Source: CAD feature listing. Evaluate the final solid. Frame: model axes, mm. A direction names the side the tool comes from. Give positions to 0.01 mm unless a question says otherwise; leave off trailing zeros. Loops run counter-clockwise (first coordinate to the right, second up) from the corner with the lowest first, then second, coordinate; pieces in that order, holes last.
```python
from build123d import *

# Parameters (mm, degrees)
SKETCH_1_W          = 40
SKETCH_1_H          = 39
EXTRUDE_1_DEPTH     = 20
SKETCH_2_W          = 20
SKETCH_2_H          = 2
EXTRUDE_2_DEPTH     = 8
SKETCH_3_W          = 20
SKETCH_3_H          = 2
EXTRUDE_3_DEPTH     = 8
CUT_EXTRUDE_3_REACH = 62.539
SKETCH_4_R          = 2
CUT_EXTRUDE_5_REACH = 62.539
SKETCH_5_R          = 2
SKETCH_7_R          = 3
EXTRUDE_5_DEPTH     = 0.5
SKETCH_9_R          = 1.5
EXTRUDE_6_DEPTH     = 5
FILLET_7_R          = 1
FILLET_8_R          = 1
FILLET_9_R          = 1
FILLET_10_R         = 1


# Read off the part's stored shape, not the designer's step: #4-40 机械螺纹 螺柱3
with BuildPart() as part:
    # 草图1 → 凸台-拉伸1 (new body)
    with BuildSketch(Plane(origin=(0, 0, 0), x_dir=(0, 0, -1), z_dir=(1, 0, 0))):
        with Locations((20, 19.5)):
            Rectangle(SKETCH_1_W, SKETCH_1_H)
    extrude(amount=EXTRUDE_1_DEPTH)

    # 草图2 → 凸台-拉伸2 (add)
    with BuildSketch(Plane.XY):
        with Locations((10, 30)):
            Rectangle(SKETCH_2_W, SKETCH_2_H)
    extrude(amount=EXTRUDE_2_DEPTH)

    # 草图3 → 凸台-拉伸3 (add)
    with BuildSketch(Plane(origin=(0, 0, -40), x_dir=(-1, 0, 0), z_dir=(0, 0, -1))):
        with Locations((-10, 30)):
            Rectangle(SKETCH_3_W, SKETCH_3_H)
    extrude(amount=EXTRUDE_3_DEPTH)

    # 草图4 → 切除-拉伸3 (cut, up to next)
    with BuildSketch(Plane(origin=(0, 31, 0), x_dir=(1, 0, 0), z_dir=(0, 1, 0)), mode=Mode.PRIVATE) as cut_extrude_3_sk1:
        with Locations(Location((5, -4, 0), (0, 0, 180))):
            Circle(SKETCH_4_R)
    cut_extrude_3_tool1 = extrude(cut_extrude_3_sk1.sketch, amount=-CUT_EXTRUDE_3_REACH, mode=Mode.PRIVATE) & part.part
    # 草图4 → 切除-拉伸3 (cut, up to next)
    with BuildSketch(Plane(origin=(0, 31, 0), x_dir=(1, 0, 0), z_dir=(0, 1, 0)), mode=Mode.PRIVATE) as cut_extrude_3_sk2:
        with Locations(Location((15, -4, 0), (0, 0, 180))):
            Circle(SKETCH_4_R)
    cut_extrude_3_tool2 = extrude(cut_extrude_3_sk2.sketch, amount=-CUT_EXTRUDE_3_REACH, mode=Mode.PRIVATE) & part.part
    add(cut_extrude_3_tool1.solids().sort_by_distance((5, 31, 4))[0], mode=Mode.SUBTRACT)
    add(cut_extrude_3_tool2.solids().sort_by_distance((15, 31, 4))[0], mode=Mode.SUBTRACT)

    # 草图5 → 切除-拉伸5 (cut, up to next)
    with BuildSketch(Plane(origin=(0, 31, 0), x_dir=(1, 0, 0), z_dir=(0, 1, 0)), mode=Mode.PRIVATE) as cut_extrude_5_sk1:
        with Locations(Location((5, 44, 0), (0, 0, 270))):
            Circle(SKETCH_5_R)
    cut_extrude_5_tool1 = extrude(cut_extrude_5_sk1.sketch, amount=-CUT_EXTRUDE_5_REACH, mode=Mode.PRIVATE) & part.part
    # 草图5 → 切除-拉伸5 (cut, up to next)
    with BuildSketch(Plane(origin=(0, 31, 0), x_dir=(1, 0, 0), z_dir=(0, 1, 0)), mode=Mode.PRIVATE) as cut_extrude_5_sk2:
        with Locations(Location((15, 44, 0), (0, 0, 270))):
            Circle(SKETCH_5_R)
    cut_extrude_5_tool2 = extrude(cut_extrude_5_sk2.sketch, amount=-CUT_EXTRUDE_5_REACH, mode=Mode.PRIVATE) & part.part
    add(cut_extrude_5_tool1.solids().sort_by_distance((5, 31, -44))[0], mode=Mode.SUBTRACT)
    add(cut_extrude_5_tool2.solids().sort_by_distance((15, 31, -44))[0], mode=Mode.SUBTRACT)

    # 草图7 → 凸台-拉伸5 (add)
    with BuildSketch(Plane(origin=(0, 39, 0), x_dir=(1, 0, 0), z_dir=(0, 1, 0))):
        with Locations(Location((10, 10, 0), (0, 0, 90))):
            Circle(SKETCH_7_R)
    extrude(amount=EXTRUDE_5_DEPTH)

    # 草图9 → 凸台-拉伸6 (add)
    with BuildSketch(Plane(origin=(0, 39, 0), x_dir=(1, 0, 0), z_dir=(0, 1, 0))):
        with Locations(Location((10, 10, 0), (0, 0, 270))):
            Circle(SKETCH_9_R)
    extrude(amount=EXTRUDE_6_DEPTH)

    # 圆角7
    fillet_7_edges = [part.edges().sort_by_distance(p)[0] for p in [
        (20, 39, -20),
        (0, 35, -40),
        (20, 35, -40),
        (20, 35, 0),
        (0, 39, -20),
        (0, 35, 0),
        (10, 39, 0),
        (10, 39, -40),
    ]]
    fillet(fillet_7_edges, radius=FILLET_7_R)

    # 圆角8
    fillet_8_edges = [part.edges().sort_by_distance(p)[0] for p in [
        (20, 30, 8),
        (0, 30, 8),
    ]]
    fillet(fillet_8_edges, radius=FILLET_8_R)

    # 圆角9
    fillet_9_edges = [part.edges().sort_by_distance(p)[0] for p in [
        (0, 30, -48),
        (20, 30, -48),
    ]]
    fillet(fillet_9_edges, radius=FILLET_9_R)

    # #4-40 机械螺纹 螺柱3 outline → #4-40 机械螺纹 螺柱3 (revolve, cut)
    with BuildSketch(Plane(origin=(10, 0, -10), x_dir=(1, 0, 0), z_dir=(0, 0, 1))):
        Polygon((1.5, 44), (1.04394, 44), (1.4224, 43.62154), (1.4224, 39.5), (1.5, 39.5), align=None)
    revolve(axis=Axis((10, 0, -10), (0, 1, 0)), mode=Mode.SUBTRACT)

    # 圆角10
    fillet_10_edges = [part.edges().sort_by_distance(p)[0] for p in [
        (20, 14.5, -40),
        (0, 14.5, 0),
        (20, 14.5, 0),
        (0, 14.5, -40),
    ]]
    fillet(fillet_10_edges, radius=FILLET_10_R)


solid = part.part
```
(1) Section A-A, the plane x = 5. Return the cut outline in (y, z), then the cut area to 3 significant figures.
A:
outline: (0, -40) - (29, -40) - (29, -42) - (31, -42) - (31, -40) - (38, -40) arc R1 ccw to (39, -39) - (39, -1) arc R1 ccw to (38, 0) - (31, 0) - (31, 2) - (29, 2) - (29, 0) - (0, 0) - close; (29, -48) - (31, -48) - (31, -46) - (29, -46) - close; (29, 6) - (31, 6) - (31, 8) - (29, 8) - close
area: 1,580 mm2
(2) Reachability of faces 1 (the flat face through (10, 34, -40)), 2 (the flat face through (10, 34, 0)), 3 (the cylindrical face through (10.66, 41.53, -8.74)) from +Z, -Z, +X, -X, +Y, -Y: full face, straight path, thin tool, end or side. Return the list, or none.
A:
face 1: -Z, +X, -X, +Y
face 2: +Z, +X, -X, +Y
face 3: +Y
(3) Section B-B, the plane z = 4. Return the cut outline in (x, y).
A:
outline: (0, 29) - (3, 29) - (3, 31) - (0, 31) - close; (7, 29) - (13, 29) - (13, 31) - (7, 31) - close; (17, 29) - (20, 29) - (20, 31) - (17, 31) - close
(4) Section C-C, the plane y = 36.5. Return the cut outline in (x, z), then the cut area to 3 significant figures.
A:
outline: (0, -39) arc R1 ccw to (1, -40) - (19, -40) arc R1 ccw to (20, -39) - (20, -1) arc R1 ccw to (19, 0) - (1, 0) arc R1 ccw to (0, -1) - close
area: 799 mm2
(5) Ray query, line 1 along X through (y, z) = (30.5, -44); line 2 along Y through (x, z) = (1.5, 5.5); line 3 along Z through (x, y) = (17, 3). Return the intervals inside material, ascending.
A:
line 1: x = 0 to 3, 7 to 13, 17 to 20
line 2: y = 29 to 31
line 3: z = -40 to 0
(6) First-contact query: pin 1 (8 mm diameter, centred on x = 8, y = 9.5, fed in from -Z); pin 2 (4.5 mm diameter, centred on x = 15, z = -44, fed in from -Y); pin 3 (4.5 mm diameter, centred on x = 13.5, z = -43.5, fed in from +Y). Flat tips, straight axial feed; report the tip coordinate or a pass-through.
A:
pin 1: stops at z = -40
pin 2: stops at y = 29
pin 3: stops at y = 31
(7) Mould query, pull axis Z, two halves, no side actions, for faces 4 (the flat face through (10, 30, 8)), 5 (the cylindrical face through (17, 30, -44)), 6 (the flat face through (10, 0, -20)). Classes: pulls with the +Z half, pulls with the -Z half, needs draft (parallel to the pull), parting line crosses it, or undercut.
A:
face 4: pulls with the +Z half
face 5: undercut
face 6: needs draft
(8) Section D-D, the plane x = 2. Return the cut outline in (y, z).
A:
outline: (0, -40) - (29, -40) - (29, -48) - (31, -48) - (31, -40) - (38, -40) arc R1 ccw to (39, -39) - (39, -1) arc R1 ccw to (38, 0) - (31, 0) - (31, 8) - (29, 8) - (29, 0) - (0, 0) - close
